Geometry: final body of the model. Coordinates: model frame, mm. Face numbers are marked on the shaded views. A direction names the side the tool comes from. Give positions to 0.01 mm unless a question says otherwise; leave off trailing zeros. Write each loop counter-clockwise with the first axis right and the second up, starting at its lowest first coordinate (ties: lowest second). Pieces come first, ordered by that corner, then holes. Notation, with made-up numbers: M 13,-21 L 28,-21 A22 ccw 28,-14 Z; hole C 0.5,-24 d5. An arc over 180 degrees is marked long. Use one line per item in the form item = value. Start each with the question number.
Item 1: Contact query for flat-ended pins moving along their axis: P1, Ø4, axis at y = 57, z = -23, coming from the +X side; P2, Ø8, axis at x = 8.5, z = -35.5, coming from the -Y side; P3, Ø3, axis at x = -57.5, z = -37, coming from the +Y side. Output: stop coordinate, or through.
Item 2: Material intervals for line 1 along Z through (x, y) = (-44.5, 51.5); line 2 along X through (y, z) = (8, -56); line 3 along Y through (x, z) = (-38, -11.5), sorted ascending. Write a range as from..to.
Item 3: Access query for the marked faces 5, 6 and 7. Directions: +Z, -Z, +X, -X, +Y, -Y. A direction counts if a zero-diameter tool reaches every point of the face in a straight line with its end or side. Return the directions, or none.
Item 4: Pull-direction query (Z, two-part tool) for the marked faces 1, 2, 3 and 4; classes: released by +Z, released by -Z, zero draft, split by the parting line, or undercut.
Item 5: Section query B-B on x = -39. Return loops of the section in (y, z), then the cut area to 3 significant figures.
Item 6: Section query A-A on y = 59.5. Return loops of the section in (x, z).
Item 7: Section query C-C on z = -88. Return loops of the section in (x, y), then the cut area to 3 significant figures.
Item 8: Section query D-D on y = 49. Return loops of the section in (x, z), then the cut area to 3 significant figures.
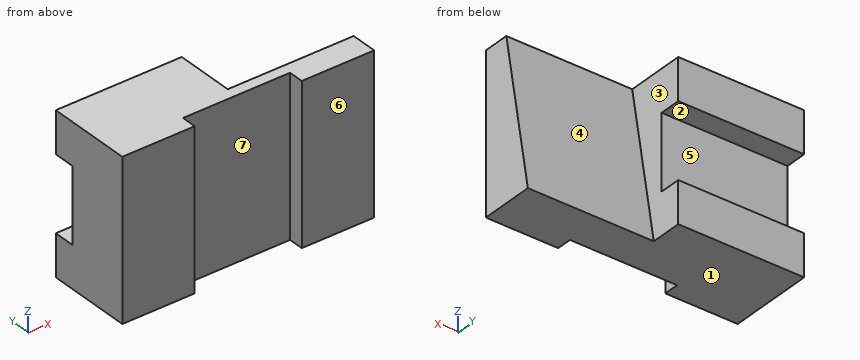
from build123d import *

# Parameters (mm, degrees)
BOSS_EXTRUDE3_DEPTH     = 100
BOSS_EXTRUDE4_DEPTH     = 100
CUT_EXTRUDE1_DEPTH      = 174.922396488
CUT_EXTRUDE1_DEPTH_BACK = 125


with BuildPart() as part:
    # Sketch3 → Boss-Extrude3 (new body)
    with BuildSketch(Plane(origin=(0, 0, 0), x_dir=(0, 0, -1), z_dir=(1, 0, 0))):
        Polygon((0, 68), (0, 0), (125, 0), (125, 68), (92, 68), (92, 51), (33, 51), (33, 68), align=None)
    extrude(amount=-BOSS_EXTRUDE3_DEPTH)

    # Sketch3_3 → Boss-Extrude4 (add)
    with BuildSketch(Plane(origin=(0, 0, 0), x_dir=(0, 0, -1), z_dir=(1, 0, 0))):
        Polygon((125, 43), (0, 20.959127411), (0, 0), (125, 0), align=None)
    extrude(amount=BOSS_EXTRUDE4_DEPTH)

    # Sketch4 → Cut-Extrude1 (cut, two sides: drawn at the far end of the back side and taken through both)
    with BuildSketch(Plane.XY.offset(-CUT_EXTRUDE1_DEPTH_BACK)):
        Polygon((-42.5, -325.78632016), (-42.5, 0), (-42.5, 12), (42.5, 12), (42.5, 0), (42.5, -325.78632016), (42.5, -977.358960479), (-42.5, -977.358960479), align=None)
    extrude(amount=CUT_EXTRUDE1_DEPTH + CUT_EXTRUDE1_DEPTH_BACK, mode=Mode.SUBTRACT)


solid = part.part
Answer sheet:
q1.P1 = 0
q1.P2 = 12
q1.P3 = 51
q2.line_1 = -125..-92, -33..0
q2.line_2 = -100..-42.5, 42.5..100
q2.line_3 = 12..68
q3.face_5 = +X, -X, +Y
q3.face_6 = +Z, -Z, +X, -X, -Y
q3.face_7 = +Z, -Z, -Y
q4.face_1 = released by -Z
q4.face_2 = undercut
q4.face_3 = zero draft
q4.face_4 = released by +Z
q5.outline = M 12,-125 L 68,-125 L 68,-92 L 51,-92 L 51,-33 L 68,-33 L 68,0 L 12,0 Z
q5.area = 6,000 mm2
q6.outline = M -100,-125 L 0,-125 L 0,-92 L -100,-92 Z; M -100,-33 L 0,-33 L 0,0 L -100,0 Z
q7.outline = M -100,0 L -42.5,0 L -42.5,12 L 42.5,12 L 42.5,0 L 100,0 L 100,36.48 L 0,36.48 L 0,51 L -100,51 Z
q7.area = 7,730 mm2
q8.outline = M -100,-125 L 0,-125 L 0,0 L -100,0 Z
q8.area = 12,500 mm2
